Could you check a few things on this model? Use its own coordinates, in mm. Face numbers are marked on the shaded views. A direction names the side the tool comes from. Coordinates: 2 decimals unless noted, no trailing zeros. Write each loop counter-clockwise with the first axis right and the second up, starting at its lowest first coordinate (ties: lowest second). Pieces come first, ordered by that corner, then holes.
Item 1: Which directions (+Z, -Z, +X, -X, +Y, -Y) give clear straight access to the entire face, cutting with the end or side of a thin tool? Please do the marked faces 1 and 2.
Item 2: I want a section at A-A on x = 37.5. Please give me the cut outline in (y, z), then the cut area to 3 significant figures.
Item 3: For P1, Ø7.5, axis at y = 17, z = 42.5, coming from the -X side; P2, Ø1, axis at x = -6.5, z = 39.5, coming from the +Y side; P3, Ø1.5, axis at x = -38.5, y = 12, coming from the +Z side; P4, Ø5, axis at x = 23, z = 11.5, coming from the -Y side, each with a flat end and sliding along its axis, tell me the tip position at first contact or that it passes through.
Item 4: I want a section at C-C on z = 42. State how many separate pieces and enclosed holes the cut face has, then the cut area to 3 significant figures.
Item 5: Thinking about a two-plate mould opening in X: for the marked faces 3, 4, 5 and 6, which applies, +X half, -X half, draft (parallel to the pull), parting line (faces both ways), or undercut?
Item 6: If I drill on probe 1 along Z at (x, y) = (3, 2.65); probe 2 along Z at (x, y) = (45, 18); probe 3 along X at (y, z) = (2.8, 29), over which ranges is the centre line in solid material (lowest first)?
Item 7: I want a section at D-D on x = -2.3. Please give me the cut outline in (y, z), then the cut area to 3 significant figures.
from build123d import *

# Parameters (mm, degrees)
SKETCH1_W                   = 97
SKETCH1_H                   = 99
BOSS_EXTRUDE1_DEPTH         = 36
SKETCH2_W                   = 96
SKETCH2_H                   = 35
CUT_EXTRUDE1_DEPTH          = 16
BOSS_EXTRUDE2_DEPTH         = 15
SKETCH4_R                   = 1.75
BOSS_EXTRUDE3_DEPTH         = 25
M3_TAPPED_HOLE1_D           = 2.5
M3_TAPPED_HOLE1_DEPTH       = 4.5
M3_TAPPED_HOLE1_CSINK_D     = 3.05
M3_TAPPED_HOLE1_CSINK_ANGLE = 90
M3_TAPPED_HOLE1_TIP         = 0.751075774
M3_TAPPED_HOLE2_D           = 2.5
M3_TAPPED_HOLE2_DEPTH       = 4.5
M3_TAPPED_HOLE2_CSINK_D     = 3.05
M3_TAPPED_HOLE2_CSINK_ANGLE = 90
M3_TAPPED_HOLE2_TIP         = 0.751075774


with BuildPart() as part:
    # Sketch1 → Boss-Extrude1 (new body)
    with BuildSketch(Plane(origin=(0, 0, 0), x_dir=(1, 0, 0), z_dir=(0, 1, 0))):
        Rectangle(SKETCH1_W, SKETCH1_H)
    extrude(amount=BOSS_EXTRUDE1_DEPTH)

    # Sketch2 → Cut-Extrude1 (cut)
    with BuildSketch(Plane.XY.offset(49.5)):
        with Locations((-0.5, 18.5)):
            Rectangle(SKETCH2_W, SKETCH2_H)
    extrude(amount=-CUT_EXTRUDE1_DEPTH, mode=Mode.SUBTRACT)

    # Sketch3 → Boss-Extrude2 (add)
    with BuildSketch(Plane.XY.offset(33.5)):
        Polygon((-35.5, 1), (12.3, 1), (12.3, 23), (11, 23), (11, 14), (3, 14), (3, 23), (1.7, 23), (1.7, 14), (-6.3, 14), (-6.3, 23), (-7.6, 23), (-7.6, 14), (-15.6, 14), (-15.6, 23), (-16.9, 23), (-16.9, 14), (-24.9, 14), (-24.9, 23), (-26.2, 23), (-26.2, 14), (-34.2, 14), (-34.2, 23), (-35.5, 23), align=None)
    extrude(amount=BOSS_EXTRUDE2_DEPTH)

    # Sketch4 → Boss-Extrude3 (add)
    with BuildSketch(Plane.XY.offset(33.5)):
        with Locations((-30.2, 16.5)):
            Circle(SKETCH4_R)
        with Locations((-20.9, 16.5)):
            Circle(SKETCH4_R)
        with Locations((-11.6, 16.5)):
            Circle(SKETCH4_R)
        with Locations((-2.3, 16.5)):
            Circle(SKETCH4_R)
        with Locations((7, 16.5)):
            Circle(SKETCH4_R)
    extrude(amount=BOSS_EXTRUDE3_DEPTH)

    # M3 Tapped Hole1
    with Locations(Plane(origin=(48.5, 0, 0), x_dir=(0, 0, -1), z_dir=(1, 0, 0))):
        with Locations((-31.5, 18), (42.5, 18)):
            CounterSinkHole(M3_TAPPED_HOLE1_D / 2, M3_TAPPED_HOLE1_CSINK_D / 2, depth=M3_TAPPED_HOLE1_DEPTH, counter_sink_angle=M3_TAPPED_HOLE1_CSINK_ANGLE)
            with Locations((0, 0, -(M3_TAPPED_HOLE1_DEPTH + M3_TAPPED_HOLE1_TIP / 2))):  # 118° drill point
                Cone(0, M3_TAPPED_HOLE1_D / 2, M3_TAPPED_HOLE1_TIP, mode=Mode.SUBTRACT)

    # M3 Tapped Hole2
    with Locations(Plane(origin=(0, 0, 0), x_dir=(-1, 0, 0), z_dir=(0, -1, 0))):
        with Locations((-3, -29), (-3, 26)):
            CounterSinkHole(M3_TAPPED_HOLE2_D / 2, M3_TAPPED_HOLE2_CSINK_D / 2, depth=M3_TAPPED_HOLE2_DEPTH, counter_sink_angle=M3_TAPPED_HOLE2_CSINK_ANGLE)
            with Locations((0, 0, -(M3_TAPPED_HOLE2_DEPTH + M3_TAPPED_HOLE2_TIP / 2))):  # 118° drill point
                Cone(0, M3_TAPPED_HOLE2_D / 2, M3_TAPPED_HOLE2_TIP, mode=Mode.SUBTRACT)


solid = part.part
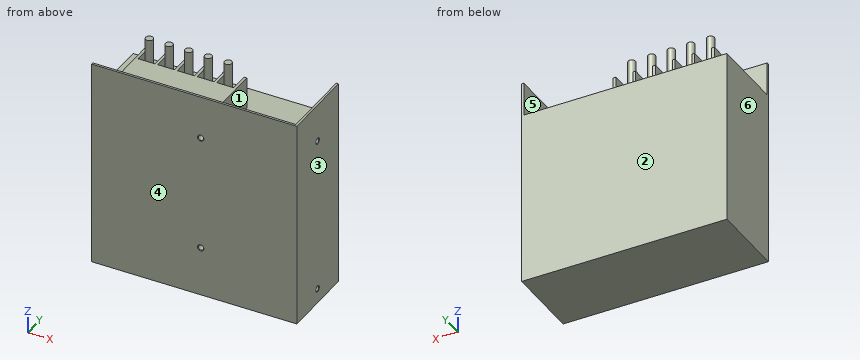
Response values:
1. face 1: +Z, +Y
1. face 2: +Z, -Z, +X, -X, +Y
2. outline: (0, -49.5) - (36, -49.5) - (36, 33.5) - (1, 33.5) - (1, 49.5) - (0, 49.5) - close
2. area: 3,000 mm2
3. P1: stops at x = -35.5
3. P2: stops at y = 23
3. P3: stops at z = 33.5
3. P4: stops at y = 0
4. separate pieces: 6
4. enclosed holes: 0
4. area: 872 mm2
5. face 3: +X half
5. face 4: draft
5. face 5: undercut
5. face 6: -X half
6. probe 1: z = -49.5 to -27.25, -24.75 to 27.75, 30.25 to 48.5
6. probe 2: z = -49.5 to -43.75, -41.25 to 30.25, 32.75 to 33.5
6. probe 3: x = -48.5 to 1.75, 4.25 to 48.5
7. outline: (0, -49.5) - (36, -49.5) - (36, 33.5) - (18.25, 33.5) - (18.25, 58.5) - (14.75, 58.5) - (14.75, 33.5) - (14, 33.5) - (14, 48.5) - (1, 48.5) - (1, 49.5) - (0, 49.5) - close
7. area: 3,290 mm2
